```python
from build123d import *

# Parameters (mm, degrees)
BOSS_EXTRUDE1_DEPTH = 4
SKETCH3_R           = 1.427241696
CUT_EXTRUDE1_DEPTH  = 62.578957395
SKETCH4_W           = 8
SKETCH4_H           = 8
BOSS_EXTRUDE3_DEPTH = 105
CUT_EXTRUDE2_REACH  = 131.405
SKETCH5_R           = 1.775
SKETCH6_R           = 1.775
CUT_EXTRUDE3_DEPTH  = 117.867981735
BOSS_EXTRUDE4_DEPTH = 8
BOSS_EXTRUDE5_DEPTH = 8


with BuildPart() as part:
    # Sketch1 → Boss-Extrude1 (new body)
    with BuildSketch(Plane(origin=(0, 0, 0), x_dir=(1, 0, 0), z_dir=(0, 1, 0))):
        Polygon((-36.424634211, -27.554537751), (-7.424634211, -27.554537751), (11.075365789, -27.554537751), (11.075365789, 8.445462249), (-7.424634211, 8.445462249), (-36.424634211, 8.445462249), (-54.924634211, 8.445462249), (-54.924634211, -27.554537751), align=None)
        with BuildLine():
            Line((-22.924634211, -4.263035129), (-20.924634211, -4.263035129))
            ThreePointArc((-20.924634211, -4.263035129), (7.075365789, -9.554537751), (-20.924634211, -14.846040373))
            Line((-20.924634211, -14.846040373), (-22.924634211, -14.846040373))
            ThreePointArc((-22.924634211, -14.846040373), (-50.924634211, -9.554537751), (-22.924634211, -4.263035129))
        make_face(mode=Mode.SUBTRACT)
    extrude(amount=BOSS_EXTRUDE1_DEPTH)

    # Sketch3 → Cut-Extrude1 (cut, through all)
    with BuildSketch(Plane.XZ):
        with Locations(Location((-21.924634211, -1.445462249, 0), (0, 0, 270))):
            Circle(SKETCH3_R)
        with Locations(Location((-21.924634211, 20.554537751, 0), (0, 0, 270))):
            Circle(SKETCH3_R)
    extrude(amount=-CUT_EXTRUDE1_DEPTH, mode=Mode.SUBTRACT)

    # Sketch4 → Boss-Extrude3 (add)
    with BuildSketch(Plane.XZ):
        with Locations((-21.924634211, -12.445462249)):
            Rectangle(SKETCH4_W, SKETCH4_H)
        with Locations((-21.924634211, 31.554537751)):
            Rectangle(SKETCH4_W, SKETCH4_H)
    extrude(amount=-BOSS_EXTRUDE3_DEPTH)

    # Cut-Extrude2: up to this face of the body (flat: up to its plane)
    cut_extrude2_end = Plane(part.part.faces().sort_by_distance((-21.924634211, 52.5, -16.445462249))[0])
    # Sketch5 → Cut-Extrude2 (cut, up to the picked face)
    with BuildSketch(Plane.XY.offset(35.554537751), mode=Mode.PRIVATE) as cut_extrude2_sk1:
        with Locations((-21.924634211, 99)):
            Circle(SKETCH5_R)
    cut_extrude2_tool1 = split(extrude(cut_extrude2_sk1.sketch, amount=-CUT_EXTRUDE2_REACH, mode=Mode.PRIVATE), bisect_by=cut_extrude2_end, keep=Keep.BOTH, mode=Mode.PRIVATE)
    add(cut_extrude2_tool1.solids().sort_by(Axis((-21.924634, 99, 35.554538), (0, 0, -1)))[0], mode=Mode.SUBTRACT)

    # Sketch6 → Cut-Extrude3 (cut, through all)
    with BuildSketch(Plane(origin=(-17.924634211, 0, 0), x_dir=(0, 0, -1), z_dir=(1, 0, 0))):
        with Locations((-31.554537751, 91.839494298)):
            Circle(SKETCH6_R)
        with Locations((12.445462249, 91.839494298)):
            Circle(SKETCH6_R)
    extrude(amount=-CUT_EXTRUDE3_DEPTH, mode=Mode.SUBTRACT)

    # Sketch7 → Boss-Extrude4 (add)
    with BuildSketch(Plane.XY.offset(27.554537751)):
        Polygon((-45.257967544, 4), (-25.924634211, 12), (-25.924634211, 0), (-54.924634211, 0), (-54.924634211, 4), align=None)
        Polygon((-17.924634211, 0), (-17.924634211, 12), (1.408699123, 4), (11.075365789, 4), (11.075365789, 0), align=None)
    extrude(amount=BOSS_EXTRUDE4_DEPTH)

    # Sketch8 → Boss-Extrude5 (add)
    with BuildSketch(Plane(origin=(0, 0, -8.445462249), x_dir=(-1, 0, 0), z_dir=(0, 0, -1))):
        Polygon((-11.075365789, 0), (-11.075365789, 4), (-1.408699123, 4), (17.924634211, 12), (17.924634211, 0), align=None)
        Polygon((25.924634211, 12), (45.257967544, 4), (54.924634211, 4), (54.924634211, 0), (25.924634211, 0), align=None)
    extrude(amount=BOSS_EXTRUDE5_DEPTH)


solid = part.part
```
Part model, mm, in its own coordinate system. A direction names the side the tool comes from. Round coordinates to 2 decimals unless told otherwise and drop trailing zeros. Write each loop counter-clockwise with the first axis right and the second up, starting at its lowest first coordinate (ties: lowest second). Pieces come first, ordered by that corner, then holes. Notation, with made-up numbers: M 77.25,24 L 91.25,24 A25 ccw 91.25,37 Z; hole C 11.25,74.25 d6. An arc over 180 degrees is marked long. One line per question, with ' | ' between items.
(1) Two-plate mould, pull along X, no slides. Class faces 3 (the face through (-25.925, 58, 31)), 4 (the face through (-22, 47, 27.555)), 5 (the face through (-21.5, 1.97, 19.19)), 6 (the face through (-22.16, 100.76, 31.61)): released by +X, released by -X, zero draft, split by the parting line, or undercut.
Answer key:
face 3: released by -X | face 4: zero draft | face 5: undercut | face 6: undercut
(2) Saw through at B-B on x = -4. Write the cut outline in (y, z), then the cut area to 3 significant figures.
Answer key:
outline: M 0,-16.45 L 6.24,-16.45 L 6.24,-8.45 L 4,-8.45 L 4,-4.54 L 0,-4.54 Z; M 0,23.64 L 4,23.64 L 4,27.55 L 6.24,27.55 L 6.24,35.55 L 0,35.55 Z | area: 131 mm^2
(3) 3-axis set-ups, long thin cutter, end or side, ignore diameter. For faces 1 (the face through (-21.9, 90.1, -12.1)), 2 (the face through (-17.925, 58, 31)): which of +Z, -Z, +X, -X, +Y, -Y reach the whole face in a straight line?
Answer key:
face 1: +X, -X | face 2: +Z, -Z, +X, +Y
(4) Probe line 1 along Z through (x, y) = (-23, 78); line 2 along Y through (x, z) = (-20.5, 33); line 3 along Y through (x, z) = (4.5, 29.5). List the from-to ranges inside material, lowest first.
Answer key:
line 1: z = -16.45 to -8.45, 27.55 to 35.55 | line 2: y = 0 to 90.81, 92.87 to 97.94, 100.06 to 105 | line 3: y = 0 to 4
(5) Saw through at D-D on z = 6. Write the cut outline in (x, y), then the cut area to 3 significant figures.
Answer key:
outline: M -54.92,0 L -50.48,0 L -50.48,4 L -54.92,4 Z; M 6.63,0 L 11.08,0 L 11.08,4 L 6.63,4 Z | area: 35.5 mm^2
(6) Pin check, flat tips, straight feed: pin 1 (9 mm diameter, centred on y = 71.5, z = 30.5, fed in from -X); pin 2 (1.7 mm diameter, centred on x = -21.92, z = 20.55, fed in from +Y); pin 3 (4 mm diameter, centred on y = 64.5, z = -12, fed in from +X); pin 4 (5.5 mm diameter, centred on x = -21.92, y = 99, fed in from +Z). Stop position of each tip, or through.
Answer key:
pin 1: stops at x = -25.92 | pin 2: passes through | pin 3: stops at x = -17.92 | pin 4: stops at z = 35.55
(7) Saw through at A-A on y = 82. Write the cut outline in (x, z), then the cut area to 3 significant figures.
Answer key:
outline: M -25.92,-16.45 L -17.92,-16.45 L -17.92,-8.45 L -25.92,-8.45 Z; M -25.92,27.55 L -17.92,27.55 L -17.92,35.55 L -25.92,35.55 Z | area: 128 mm^2
(8) Saw through at C-C on y = 99. Write the cut outline in (x, z).
Answer key:
outline: M -25.92,-16.45 L -23.7,-16.45 L -23.7,-8.45 L -25.92,-8.45 Z; M -25.92,27.55 L -23.7,27.55 L -23.7,35.55 L -25.92,35.55 Z; M -20.15,-16.45 L -17.92,-16.45 L -17.92,-8.45 L -20.15,-8.45 Z; M -20.15,27.55 L -17.92,27.55 L -17.92,35.55 L -20.15,35.55 Z
